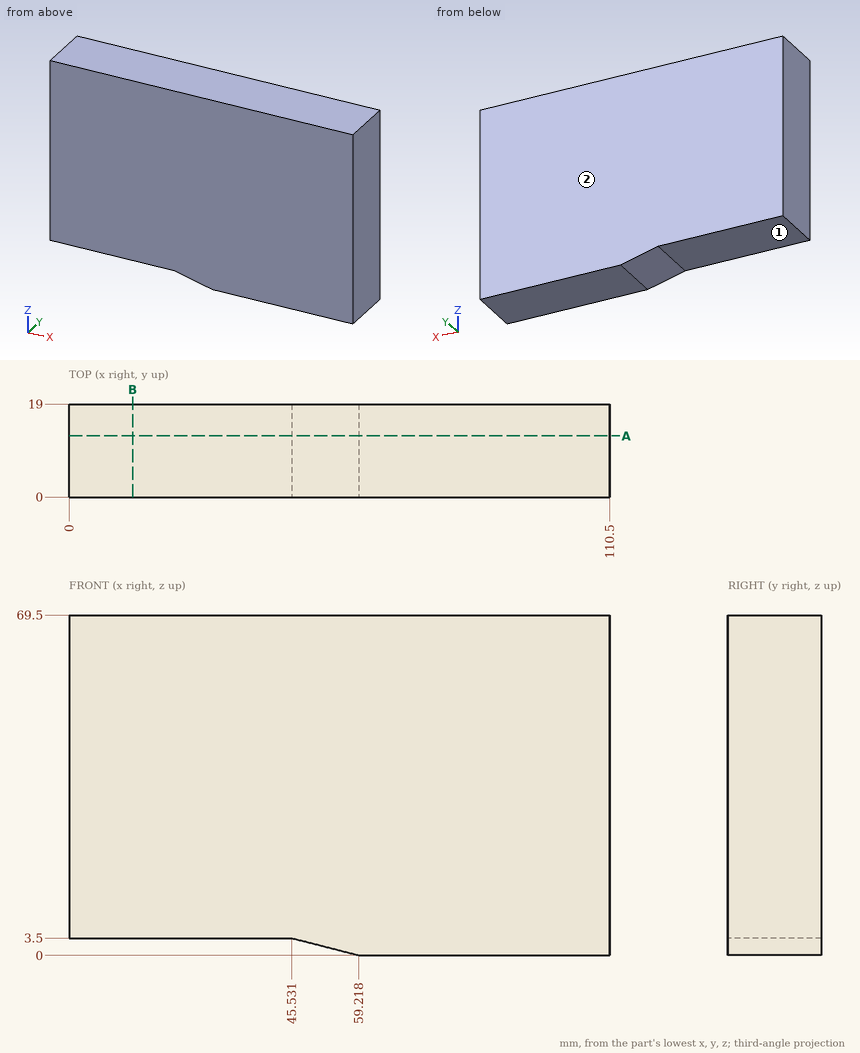
Job drawing, mm, ordinate dimensions from the low corner. One solid piece. A direction names the side the tool comes from. Give positions to 0.01 mm unless a question says otherwise; leave off trailing zeros. Write each loop counter-clockwise with the first axis right and the second up, starting at its lowest first coordinate (ties: lowest second). Pieces come first, ordered by that corner, then holes. Notation, with made-up numbers: M 65,53 L 118,53 A32 cw 118,89 Z; hole C 10,-23.5 d6. An arc over 180 degrees is marked long. One line per item, written item: value. Start each with the question number.
Q1. Saw through at A-A, the plane y = 12.5. Write the cut outline in (x, z).
Q2. Probe probe 1 along Z at (x, y) = (8, 10.5); probe 2 along Z at (x, y) = (47.5, 3.75). List the from-to ranges inside material, lowest first. Write a range as [from, to].
Q3. Saw through at B-B, the plane x = 13. Write the cut outline in (y, z).
Q4. Drop flat-ended pins along their axis: pin 1 Ø12 at (x, z) = (11.5, 45) entering from -Y; pin 2 Ø4 at (x, y) = (52.5, 3) entering from -Z; pin 3 Ø5.5 at (x, y) = (21, 5) entering from -Z; pin 4 Ø2 at (x, y) = (49, 7) entering from -Z. Give the stop position or say it passes through.
Q5. 3-axis set-ups, long thin cutter, end or side, ignore diameter. For the marked faces 1 and 2: which of +Z, -Z, +X, -X, +Y, -Y reach the whole face in a straight line?
Output values:
1. outline: M 0,3.5 L 45.53,3.5 L 59.22,0 L 110.5,0 L 110.5,69.5 L 0,69.5 Z
2. probe 1: z = [3.5, 69.5]
2. probe 2: z = [3, 69.5]
3. outline: M 0,3.5 L 19,3.5 L 19,69.5 L 0,69.5 Z
4. pin 1: stops at y = 0
4. pin 2: stops at z = 1.21
4. pin 3: stops at z = 3.5
4. pin 4: stops at z = 2.36
5. face 1: -Z, -X, +Y, -Y
5. face 2: +Z, -Z, +X, -X, +Y
